Can you work these out from the model? Positions are in its coordinate system, mm. A direction names the side the tool comes from. Coordinates: 2 decimals unless noted, no trailing zeros. Write each loop counter-clockwise with the first axis right and the second up, starting at its lowest first coordinate (ties: lowest second). Pieces come first, ordered by that corner, then holes.
```python
from build123d import *

# Parameters (mm, degrees)
F0_R     = 10.85215
F1_DEPTH = 88.9
F3_D     = 14.732
F5_DEPTH = 6.35
F7_D     = 5.842
F8_R     = 5.715
F9_DEPTH = 2.54


with BuildPart() as f1:
    # F0 (on Front) → F1 (new body)
    with BuildSketch(Plane.XZ):
        Circle(F0_R)
    extrude(amount=F1_DEPTH)

    # F3 (through all)
    with Locations(Plane.XZ.offset(88.9)):
        with Locations((0, 0)):
            Hole(F3_D / 2)

    # F4 (on Front) → F5 (join)
    with BuildSketch(Plane.XZ):
        Polygon((0, 0), (0, 34.925), (-38.1, 34.925), (-38.1, -9.525), (0, -34.925), align=None)
        Polygon((38.1, 34.925), (0, 34.925), (0, 0), (0, -34.925), (38.1, -9.525), align=None)
    extrude(amount=-F5_DEPTH)

    # F7 (through all)
    with Locations(Plane(origin=(0, 6.35, 0), x_dir=(-1, 0, 0), z_dir=(0, 1, 0))):
        with Locations((-19.05, 26.55945), (19.05, 26.55945), (19.05, -11.54055), (-19.05, -11.54055)):
            Hole(F7_D / 2)

    # F8 (on face) → F9 (cut)
    with BuildSketch(Plane.XZ):
        with Locations((-19.05, 26.55945)):
            Circle(F8_R)
        with Locations((19.05, 26.55945)):
            Circle(F8_R)
        with Locations((-19.05, -11.54055)):
            Circle(F8_R)
        with Locations((19.05, -11.54055)):
            Circle(F8_R)
    extrude(amount=-F9_DEPTH, mode=Mode.SUBTRACT)


solid = f1.part
```
1. If we section it at C-C, the plane y = -30: List the corners of the cut face in (x, z) for me, plus the area to 3 significant figures.
2. If I drill on L1, parallel to Z at x = -19.05, y = 1.35 (3 decimals); L2, parallel to Z at x = 0, y = -66; L3, parallel to Z at x = -19, y = 4 (3 decimals), over which ranges is the centre line in solid material (lowest first)?
3. We'd pull the mould along Z, two halves only. Please class faces 1 (the face through (-16.41, 1.25, 21.49)), 2 (the face through (-2.353, -43.828, -10.594)), 3 (the face through (38.1, 3, 12)): released by +Z, released by -Z, zero draft, split by the parting line, or undercut.
4. If we section it at D-D, the plane x = -9: List the corners of the cut face in (y, z) for me (3 decimals).
5. If we section it at A-A, the plane x = 19.05: List the corners of the cut face in (y, z) for me (3 decimals), plus the area to 3 significant figures.
6. Which directions (+Z, -Z, +X, -X, +Y, -Y) give clear straight access to the entire face, cutting with the end or side of a thin tool? Please do faces 4 (the face through (20.62, 4.418, -9.078)), 5 (the face through (17.81, 1.25, -17.12)).
7. If we section it at B-B, the plane z = 0: List the corners of the cut face in (x, y) for me.
8. I'm going to push flat-ended pins straight in: P1, Ø1.5, axis at x = -19.5, z = -20, coming from the -Y side; P2, Ø12, axis at x = 5.5, y = -43, coming from the -Z side; P3, Ø3, axis at y = -15, z = -5, coming from the -X side; P4, Ø3.5, axis at x = 19.05, z = -11.54, coming from the +Y side. Where does each tip first touch, or does it pass through?
Answers:
1. outline: circle Ø21.7 at (0, 0); hole circle Ø14.73 at (0, 0)
1. area: 200 mm2
2. L1: z = -22.225 to -17.256, -5.826 to 20.844, 32.274 to 34.925
2. L2: z = -10.85 to -7.37, 7.37 to 10.85
2. L3: z = -22.258 to -14.461, -8.62 to 23.639, 29.48 to 34.925
3. face 1: undercut
3. face 2: split by the parting line
3. face 3: zero draft
4. outline: (-88.9, -6.064) - (0, -6.064) - (0, -28.925) - (6.35, -28.925) - (6.35, 34.925) - (0, 34.925) - (0, 6.064) - (-88.9, 6.064) - close
5. outline: (0, -22.225) - (6.35, -22.225) - (6.35, -14.462) - (2.54, -14.462) - (2.54, -17.256) - (0, -17.256) - close; (0, -5.826) - (2.54, -5.826) - (2.54, -8.62) - (6.35, -8.62) - (6.35, 23.638) - (2.54, 23.638) - (2.54, 20.844) - (0, 20.844) - close; (0, 32.274) - (2.54, 32.274) - (2.54, 29.48) - (6.35, 29.48) - (6.35, 34.925) - (0, 34.925) - close
5. area: 260 mm2
6. face 4: +Y, -Y
6. face 5: -Y
7. outline: (-38.1, 0) - (-10.85, 0) - (-10.85, -88.9) - (-7.37, -88.9) - (-7.37, 0) - (7.37, 0) - (7.37, -88.9) - (10.85, -88.9) - (10.85, 0) - (38.1, 0) - (38.1, 6.35) - (-38.1, 6.35) - close
8. P1: stops at y = 0
8. P2: stops at z = -10.85
8. P3: stops at x = -10.27
8. P4: passes through
